Build history of the part. All positions in model axes, mm. A direction names the side the tool comes from. Coordinates: 2 decimals unless noted, no trailing zeros. Order: outer loops, then holes, each group sorted by start corner. A loop starts at its lowest first (then second) coordinate and runs counter-clockwise, first axis right, second up. Notation, with made-up numbers: (-36.75, 40) - (-15.75, 40) arc R32 ccw to (-15.75, 73) - close; hole circle Ø8 at (54.25, -14). An arc over 180 degrees is marked (long way). Return JSON: item names as keys, results as strings.
from build123d import *

# Parameters (mm, degrees)
SKETCH_1_W          = 14.5
SKETCH_1_H          = 13
EXTRUDE_1_DEPTH     = 9
EXTRUDE_2_DEPTH     = 2.5
SKETCH_3_W          = 12
SKETCH_3_H          = 7
CUT_EXTRUDE_1_DEPTH = 9.7
CUT_EXTRUDE_2_DEPTH = 6.5
SKETCH_5_W          = 7.522723779
SKETCH_5_H          = 5
CUT_EXTRUDE_3_DEPTH = 6.5
SKETCH_6_W          = 1
SKETCH_6_H          = 8
CUT_EXTRUDE_4_DEPTH = 1


with BuildPart() as part:
    # 草图1 → 凸台-拉伸1 (new body)
    with BuildSketch(Plane(origin=(0, 0, 0), x_dir=(1, 0, 0), z_dir=(0, 1, 0))):
        with Locations((1.514240506, -0.993670886)):
            Rectangle(SKETCH_1_W, SKETCH_1_H)
    extrude(amount=EXTRUDE_1_DEPTH)

    # 草图2 → 凸台-拉伸2 (add)
    with BuildSketch(Plane.XZ):
        Polygon((-5.735759494, -3.506329114), (-5.735759494, -5.506329114), (8.764240506, -5.506329114), (8.764240506, -3.506329114), (8.014240506, -3.506329114), (8.014240506, 4.493670886), (-4.985759494, 4.493670886), (-4.985759494, -3.506329114), align=None)
    extrude(amount=EXTRUDE_2_DEPTH)

    # 草图3 → 切除-拉伸1 (cut)
    with BuildSketch(Plane(origin=(0, 0, -5.506329114), x_dir=(-1, 0, 0), z_dir=(0, 0, -1))):
        with Locations((-1.514240506, 3.5)):
            Rectangle(SKETCH_3_W, SKETCH_3_H)
    extrude(amount=-CUT_EXTRUDE_1_DEPTH, mode=Mode.SUBTRACT)

    # 草图4 → 切除-拉伸2 (cut)
    with BuildSketch(Plane(origin=(0, 0, -5.506329114), x_dir=(-1, 0, 0), z_dir=(0, 0, -1))):
        Polygon((-4.514240506, 0), (1.485759494, 0), (1.485759494, -1.5), (0.235759494, -1.5), (0.235759494, -2.5), (-3.264240506, -2.5), (-3.264240506, -1.5), (-4.514240506, -1.5), align=None)
    extrude(amount=-CUT_EXTRUDE_2_DEPTH, mode=Mode.SUBTRACT)

    # 草图5 → 切除-拉伸3 (cut)
    with BuildSketch(Plane.XZ.offset(2.5)):
        with Locations((1.514240506, -1.506329114)):
            Rectangle(SKETCH_5_W, SKETCH_5_H)
    extrude(amount=-CUT_EXTRUDE_3_DEPTH, mode=Mode.SUBTRACT)

    # 草图6 → 切除-拉伸4 (cut)
    with BuildSketch(Plane.XZ.offset(2.5)):
        with Locations((-3.615759494, -0.375358935)):
            Rectangle(SKETCH_6_W, SKETCH_6_H)
        with Locations((6.644240506, -0.375358935)):
            Rectangle(SKETCH_6_W, SKETCH_6_H)
    extrude(amount=-CUT_EXTRUDE_4_DEPTH, mode=Mode.SUBTRACT)


solid = part.part
1. Mould opens along Y. For faces 1 (the flat face through (-2.247, -1, -2)), 2 (the flat face through (-4.486, 3, -1)), 3 (the flat face through (-1, -1.5, -5)), 4 (the flat face through (3, -2.5, 2)) say: pulls with the +Y half, pulls with the -Y half, needs draft (parallel to the pull), parting line crosses it, or undercut.
Check values:
{"face 1": "needs draft", "face 2": "undercut", "face 3": "undercut", "face 4": "pulls with the -Y half"}
2. Probe L1, parallel to Y at x = -1.5, z = 3; L2, parallel to X at y = 5.5, z = 4; L3, parallel to Z at x = 5, y = 6. List the from-to ranges inside material, lowest first.
Check values:
{"L1": "-2.5 to 0, 7 to 9", "L2": "-5.74 to -4.49, 7.51 to 8.76", "L3": "4.19 to 7.49"}
3. Drop flat-ended pins along their axis: pin 1 (0.8 mm diameter, centred on x = 6.5, y = -2, fed in from +Z); pin 2 (1.5 mm diameter, centred on x = 2.5, z = -3, fed in from -Y); pin 3 (5.5 mm diameter, centred on x = 4, y = 3, fed in from -Z). Give the stop position or say it passes through.
Check values:
{"pin 1": "z = 4.49", "pin 2": "y = 7", "pin 3": "z = 4.19"}
4. Cut at D-D on y = -1. Give the cut face in (x, z), plus the area to 3 significant figures.
Check values:
{"outline": "(-5.74, -5.51) - (-1.49, -5.51) - (-1.49, -4.01) - (-2.25, -4.01) - (-2.25, 0.99) - (5.28, 0.99) - (5.28, -4.01) - (4.51, -4.01) - (4.51, -5.51) - (8.76, -5.51) - (8.76, -3.51) - (8.01, -3.51) - (8.01, 4.49) - (-4.99, 4.49) - (-4.99, -3.51) - (-5.74, -3.51) - close", "area": "86.4 mm²"}
5. Cut at A-A on x = 3.75. Give the cut face in (y, z), plus the area to 4 significant figures.
Check values:
{"outline": "(-2.5, -5.51) - (-1.5, -5.51) - (-1.5, -4.01) - (-2.5, -4.01) - close; (-2.5, 0.99) - (0, 0.99) - (0, 4.19) - (7, 4.19) - (7, -5.51) - (9, -5.51) - (9, 7.49) - (0, 7.49) - (0, 4.49) - (-2.5, 4.49) - close", "area": "59.35 mm²"}
6. Cut at C-C on x = 0. Give the cut face in (y, z).
Check values:
{"outline": "(-2.5, 0.99) - (0, 0.99) - (0, 4.19) - (7, 4.19) - (7, -5.51) - (9, -5.51) - (9, 7.49) - (0, 7.49) - (0, 4.49) - (-2.5, 4.49) - close"}
7. Cut at B-B on z = -1.75. Give the cut face in (x, y), plus the area to 3 significant figures.
Check values:
{"outline": "(-5.74, 0) - (-4.99, 0) - (-4.99, -2.5) - (-4.12, -2.5) - (-4.12, -1.5) - (-3.12, -1.5) - (-3.12, -2.5) - (-2.25, -2.5) - (-2.25, 0) - (-4.49, 0) - (-4.49, 7) - (7.51, 7) - (7.51, 0) - (5.28, 0) - (5.28, -2.5) - (6.14, -2.5) - (6.14, -1.5) - (7.14, -1.5) - (7.14, -2.5) - (8.01, -2.5) - (8.01, 0) - (8.76, 0) - (8.76, 9) - (-5.74, 9) - close", "area": "58.2 mm²"}
8. Tool access for faces 5 (the flat face through (8.014, -1, 0)), 6 (the flat face through (2, 7, -1)), 7 (the flat face through (-3.6, -2, -4.375)), 8 (the flat face through (-0.236, -2, -5)): list every direction of +Z, -Z, +X, -X, +Y, -Y with a clear straight run to the whole face (end or side of a thin tool).
Check values:
{"face 5": "+Z, +X, -Y", "face 6": "-Z", "face 7": "-Y", "face 8": "-Z, -Y"}
